The model under review builds one solid part; all positions refer to its coordinate system, in mm. Face numbers are marked on the shaded views. A direction names the side the tool comes from. Coordinates: 2 decimals unless noted, no trailing zeros. Write each loop counter-clockwise with the first axis right and the second up, starting at its lowest first coordinate (ties: lowest second). Pieces come first, ordered by that corner, then holes. Notation, with made-up numbers: M 58,-35 L 79,-35 A22 ccw 79,-14 Z; hole C -11.5,-26 d5. An arc over 180 degrees is marked long. Answer as a JSON object with one key per item and string values.
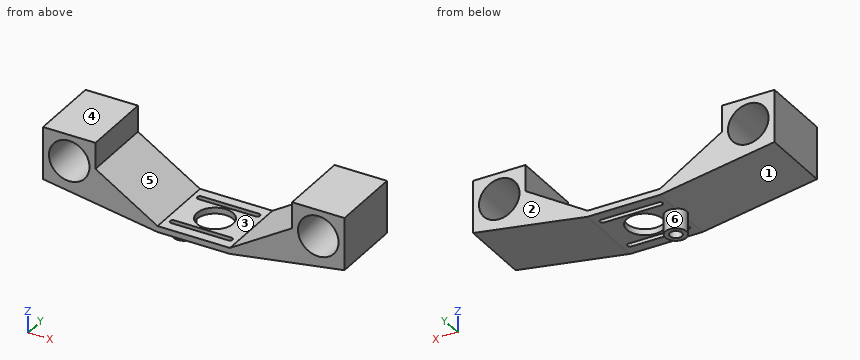
```python
from build123d import *

# Parameters (mm, degrees)
SKETCH2_R           = 13.45
BOSS_EXTRUDE1_DEPTH = 48
SKETCH4_R           = 12
CUT_EXTRUDE1_DEPTH  = 48
SKETCH5_R           = 7
SKETCH5_R_2         = 4
BOSS_EXTRUDE2_DEPTH = 2
BOSS_EXTRUDE3_START = 13
SKETCH6_R           = 7
SKETCH6_R_2         = 4
BOSS_EXTRUDE3_DEPTH = 13


with BuildPart() as part:
    # Sketch2 → Boss-Extrude1 (new body)
    with BuildSketch(Plane(origin=(0, 0, 0), x_dir=(1, 0, 0), z_dir=(0, 1, 0))):
        Polygon((-17.4, -17.4), (17.4, -17.4), (17.4, 0), (58.6, 25.6), (82.6, 25.6), (82.6, 29.6), (58.6, 29.6), (-17.4, 17.4), align=None)
        with Locations(Location((0, 0, 0), (0, 0, 270))):
            Circle(SKETCH2_R, mode=Mode.SUBTRACT)
    boss_extrude1 = extrude(amount=BOSS_EXTRUDE1_DEPTH)

    # Mirror1: Boss-Extrude1 across plane
    add(boss_extrude1.mirror(Plane(origin=(82.6, 0, 0), x_dir=(0, 0, 1), z_dir=(1, 0, 0))))

    # Sketch4 → Cut-Extrude1 (cut)
    with BuildSketch(Plane(origin=(0, 0, -29.6), x_dir=(-1, 0, 0), z_dir=(0, 0, -1))):
        with Locations((-82.6, 24)):
            Circle(SKETCH4_R)
        with BuildLine():
            Line((-101.6, 10.3), (-63.6, 10.3))
            ThreePointArc((-63.6, 10.3), (-61.85, 8.55), (-63.6, 6.8))
            Line((-63.6, 6.8), (-101.6, 6.8))
            ThreePointArc((-101.6, 6.8), (-103.35, 8.55), (-101.6, 10.3))
        make_face()
        with BuildLine():
            Line((-101.6, 37.7), (-63.6, 37.7))
            ThreePointArc((-63.6, 37.7), (-61.85, 39.45), (-63.6, 41.2))
            Line((-63.6, 41.2), (-101.6, 41.2))
            ThreePointArc((-101.6, 41.2), (-103.35, 39.45), (-101.6, 37.7))
        make_face()
    extrude(amount=-CUT_EXTRUDE1_DEPTH, mode=Mode.SUBTRACT)

    # Sketch5 → Boss-Extrude2 (add)
    with BuildSketch(Plane(origin=(0, 0, -29.6), x_dir=(-1, 0, 0), z_dir=(0, 0, -1))):
        with Locations((-62.1, 24)):
            Circle(SKETCH5_R)
        with Locations((-62.1, 24)):
            Circle(SKETCH5_R_2, mode=Mode.SUBTRACT)
    extrude(amount=-BOSS_EXTRUDE2_DEPTH)

    # Sketch6 → Boss-Extrude3 (add)
    with BuildSketch(Plane(origin=(0, 0, -29.6), x_dir=(-1, 0, 0), z_dir=(0, 0, -1)).offset(BOSS_EXTRUDE3_START)):
        with Locations((-62.1, 24)):
            Circle(SKETCH6_R)
        with Locations((-62.1, 24)):
            Circle(SKETCH6_R_2, mode=Mode.SUBTRACT)
    extrude(amount=-BOSS_EXTRUDE3_DEPTH)


solid = part.part
```
(1) Wall thickness on line 1 along X through (y, z) = (35.5, 0); line 2 along Y through (x, z) = (82.6, -27.6); line 3 along X through (y, z) = (24, -37.5): over which ranges is each line inside the solid? List them lowest first. Write a range as from..to.
Results list:
{"line 1": "-17.4..-13.45, 13.45..17.4, 147.8..151.75, 178.65..182.6", "line 2": "0..6.8, 10.3..12, 36..37.7, 41.2..48", "line 3": "55.1..58.1, 66.1..69.1"}
(2) Add section B-B on x = 82.6. Give the boundary of the cut face in (y, z).
Results list:
{"outline": "M 0,-29.6 L 6.8,-29.6 L 6.8,-25.6 L 0,-25.6 Z; M 10.3,-29.6 L 12,-29.6 L 12,-25.6 L 10.3,-25.6 Z; M 36,-29.6 L 37.7,-29.6 L 37.7,-25.6 L 36,-25.6 Z; M 41.2,-29.6 L 48,-29.6 L 48,-25.6 L 41.2,-25.6 Z"}
(3) Add section C-C on z = -22. Give the boundary of the cut face in (x, y).
Results list:
{"outline": "M 11.26,0 L 52.81,0 L 52.81,48 L 11.26,48 Z; M 112.39,0 L 153.94,0 L 153.94,48 L 112.39,48 Z"}
(4) Draft analysis for pull direction X (two halves, no side actions). For the marked faces 1, 2 and 3, state which applies: released by +X, released by -X, zero draft, split by the parting line, or undercut.
Results list:
{"face 1": "released by -X", "face 2": "zero draft", "face 3": "undercut"}
(5) For the marked faces 4, 5 and 6, list the 3-axis set-ups (+Z, -Z, +X, -X, +Y, -Y) from which the entire face can be reached by the end or side of a thin tool; tool diameter is ignored.
Results list:
{"face 4": "+Z, +X, -X, +Y, -Y", "face 5": "+Z, +Y, -Y", "face 6": "-Z"}
(6) Add section A-A on y = 8.55. Give the boundary of the cut face in (x, z).
Results list:
{"outline": "M -17.4,-17.4 L 58.6,-29.6 L 61.85,-29.6 L 61.85,-25.6 L 58.6,-25.6 L 17.4,0 L 17.4,17.4 L -17.4,17.4 Z; M 103.35,-29.6 L 106.6,-29.6 L 182.6,-17.4 L 182.6,17.4 L 147.8,17.4 L 147.8,0 L 106.6,-25.6 L 103.35,-25.6 Z; hole C 0,0 d26.9; hole C 165.2,0 d26.9"}
(7) For pin 1 Ø21.5 at (x, y) = (82.6, 24) entering from -Z; pin 2 Ø8 at (x, y) = (105.5, 12.5) entering from -Z; pin 3 Ø5 at (x, y) = (124, 14) entering from +Z; pin 4 Ø6 at (x, y) = (143.5, 26) entering from -Z, all flat-tipped, find the tip position at first contact; note any pin that passes through.
Results list:
{"pin 1": "through", "pin 2": "z = -29.6", "pin 3": "z = -13.23", "pin 4": "z = -24.16"}
(8) Add section D-D on y = 24. Give the boundary of the cut face in (x, z).
Results list:
{"outline": "M -17.4,-17.4 L 55.1,-29.04 L 55.1,-42.6 L 58.1,-42.6 L 58.1,-29.52 L 58.6,-29.6 L 66.1,-29.6 L 66.1,-42.6 L 69.1,-42.6 L 69.1,-29.6 L 70.6,-29.6 L 70.6,-25.6 L 58.6,-25.6 L 17.4,0 L 17.4,17.4 L -17.4,17.4 Z; M 94.6,-29.6 L 106.6,-29.6 L 182.6,-17.4 L 182.6,17.4 L 147.8,17.4 L 147.8,0 L 106.6,-25.6 L 94.6,-25.6 Z; hole C 0,0 d26.9; hole C 165.2,0 d26.9"}
